```python
from build123d import *

# Parameters (mm, degrees)
BOSS_EXTRUDE1_DEPTH = 25
SKETCH2_R           = 1.5
BOSS_EXTRUDE2_DEPTH = 7
SKETCH3_R           = 1.5
CUT_EXTRUDE1_DEPTH  = 7
FILLET1_R           = 1


with BuildPart() as part:
    # Sketch1 → Boss-Extrude1 (new body)
    with BuildSketch(Plane(origin=(0, 0, 0), x_dir=(1, 0, 0), z_dir=(0, 1, 0))):
        Polygon((2.214824591, -1.851454932), (2.7108193, 0.992366895), (0.495994709, 2.843821827), (-2.214824591, 1.851454932), (-2.7108193, -0.992366895), (-0.495994709, -2.843821827), align=None)
    extrude(amount=BOSS_EXTRUDE1_DEPTH)

    # Sketch2 → Boss-Extrude2 (add)
    with BuildSketch(Plane(origin=(0, 25, 0), x_dir=(1, 0, 0), z_dir=(0, 1, 0))):
        Circle(SKETCH2_R)
    extrude(amount=BOSS_EXTRUDE2_DEPTH)

    # Sketch3 → Cut-Extrude1 (cut)
    with BuildSketch(Plane.XZ):
        Circle(SKETCH3_R)
    extrude(amount=-CUT_EXTRUDE1_DEPTH, mode=Mode.SUBTRACT)

    # Fillet1
    fillet1_edges = [part.edges().sort_by_distance(p)[0] for p in [
        (-1.5, 32, 0),
    ]]
    fillet(fillet1_edges, radius=FILLET1_R)


solid = part.part
```
Can you work these out from the model? Positions are in its coordinate system, mm. A direction names the side the tool comes from. Coordinates: 2 decimals unless noted, no trailing zeros. Loops run counter-clockwise (first coordinate to the right, second up) from the corner with the lowest first, then second, coordinate; pieces in that order, holes last. Notation, with made-up numbers: (58, 73) -> (97, 73) arc R24 cw to (97, 94) -> close; hole circle Ø5 at (1, -18). An arc over 180 degrees is marked (long way). Answer as a JSON object with one key per item and string values.
1) Imagine slicing it at B-B (z = 2.3). Please give me the cut outline in (x, y).
Results:
{"outline": "(-1.15, 0) -> (0.99, 0) -> (0.99, 25) -> (-1.15, 25) -> close"}
2) For faces 1 (the face through (2.46, 12.32, 0.45)), 2 (the face through (-1.5, 3.45, 0.07)), 3 (the face through (1.2, 25, 1.2)), which set-ups out of +Z, -Z, +X, -X, +Y, -Y let a thin tool reach every point of the face, with its end or its side?
Results:
{"face 1": "+Z, +X, +Y, -Y", "face 2": "-Y", "face 3": "+Y"}
3) If I drill on line 1 (Y direction, x = -1.85, z = 0.55); line 2 (X direction, y = 2, z = -0.15); line 3 (Z direction, x = 0, y = 4.5), over which ranges is the centre line in solid material (lowest first)?
Results:
{"line 1": "y = 0 to 25", "line 2": "x = -2.51 to -1.49, 1.49 to 2.56", "line 3": "z = -2.66 to -1.5, 1.5 to 2.66"}
4) For P1, Ø2.5, axis at x = 0, z = 0, coming from the -Y side; P2, Ø1, axis at x = -1.5, z = 2, coming from the +Y side, each with a flat end and sliding along its axis, tell me the tip position at first contact or that it passes through.
Results:
{"P1": "stops at y = 7", "P2": "stops at y = 25"}
5) Imagine slicing it at A-A (y = 21.5). Please give me the cut outline in (x, z), then the cut area to 3 significant figures.
Results:
{"outline": "(-2.71, 0.99) -> (-2.21, -1.85) -> (0.5, -2.84) -> (2.71, -0.99) -> (2.21, 1.85) -> (-0.5, 2.84) -> close", "area": "21.7 mm^2"}
6) Imagine slicing it at C-C (z = -2.2). Please give me the cut outline in (x, y), then the cut area to 3 significant figures.
Results:
{"outline": "(-1.26, 0) -> (1.27, 0) -> (1.27, 25) -> (-1.26, 25) -> close", "area": "63.2 mm^2"}
7) Thinking about a two-plate mould opening in X: for faces 4 (the face through (0.84, 12.325, 2.355)), 5 (the face through (0, 7, 0)), 6 (the face through (-0.84, 12.325, -2.355)), 7 (the face through (-1.5, 27.96, -0.07)), which applies, pulls with the +X half, pulls with the -X half, needs draft (parallel to the pull), parting line crosses it, or undercut?
Results:
{"face 4": "pulls with the +X half", "face 5": "undercut", "face 6": "pulls with the -X half", "face 7": "parting line crosses it"}
